Work out the finished part from the listing and answer in its coordinate system (mm). A direction names the side the tool comes from. Give positions to 0.01 mm unless a question says otherwise; leave off trailing zeros. Write each loop counter-clockwise with the first axis right and the second up, starting at its lowest first coordinate (ties: lowest second). Pieces come first, ordered by that corner, then holes.
1) Determine the mould class of faces 1 (the face through (6, 0, 3)), 2 (the face through (0, 3.8, 8)), 3 (the face through (1.5, 0.07, -0.49)) for opening direction X: pulls with the +X half, pulls with the -X half, needs draft (parallel to the pull), parting line crosses it, or undercut.
2) Find section D-D (x = 2.5). Determine the outline of the cut face in (y, z), plus the area to 3 significant figures.
3) Find section B-B (x = 0). Determine the outline of the cut face in (y, z).
4) Given pin 1 Ø1.5 at (y, z) = (2, -1.5) entering from +X; pin 2 Ø3 at (y, z) = (3.5, 0) entering from +X; pin 3 Ø1.2 at (x, z) = (0, 8.5) entering from +Y, each flat-ended and moving along its own axis, determine where each tip first touches the part or whether it passes through.
5) Straight lines are drawn through the part: probe 1 along Y at (x, z) = (2.5, -0.25); probe 2 along X at (y, z) = (5.25, 1.5); probe 3 along Y at (x, z) = (1.5, 6.75). For each, find the intervals that lie inside material, in ascending order.
6) Find section C-C (y = 4). Determine the outline of the cut face in (x, z).
7) A tool of negligible diameter and unlimited length cuts with its end or side. For faces 4 (the face through (4, 0, 6)), 5 (the face through (4.6, 0, -0.5)), 6 (the face through (3.8, 0, 8)), 7 (the face through (-3.8, 0, 8)), 8 (the face through (0, -3.8, 8)), from which of +Z, -Z, +X, -X, +Y, -Y can it reach the whole face along a straight path? Write none if from no direction.
8) Find section A-A (z = 9.25). Determine the outline of the cut face in (x, y), plus the area to 3 significant figures.
```python
from build123d import *

# Parameters (mm, degrees)
BOSS_EXTRU_1_DEPTH      = 6
ESQUISSE2_W             = 7.6
ESQUISSE2_H             = 7.6
BOSS_EXTRU_2_DEPTH      = 4
ENL_V_MAT_EXTRU_1_DEPTH = 0.1
ESQUISSE4_R             = 1.5
ESQUISSE4_R_2           = 0.6
BOSS_EXTRU_4_DEPTH      = 1.2
ESQUISSE5_R             = 0.4
BOSS_EXTRU_5_DEPTH      = 5.2
CONG_1_R                = 0.5


with BuildPart() as part:
    # Esquisse1 → Boss.-Extru.1 (new body)
    with BuildSketch(Plane.XY):
        with BuildLine():
            Line((-5.4, 2.615339366), (-5.4, -2.615339366))
            ThreePointArc((-5.4, -2.615339366), (6, 0), (-5.4, 2.615339366))
        make_face()
    extrude(amount=BOSS_EXTRU_1_DEPTH)

    # Esquisse2 → Boss.-Extru.2 (add)
    with BuildSketch(Plane.XY.offset(6)):
        Rectangle(ESQUISSE2_W, ESQUISSE2_H)
    extrude(amount=BOSS_EXTRU_2_DEPTH)

    # Esquisse3 → Enlèv. mat.-Extru.1 (cut)
    with BuildSketch(Plane(origin=(0, 0, 0), x_dir=(-1, 0, 0), z_dir=(0, 0, -1))):
        with BuildLine():
            Line((4.8, -2.473863375), (4.8, 2.473863375))
            ThreePointArc((4.8, 2.473863375), (-5.4, 0), (4.8, -2.473863375))
        make_face()
    extrude(amount=-ENL_V_MAT_EXTRU_1_DEPTH, mode=Mode.SUBTRACT)

    # Esquisse4 → Boss.-Extru.4 (add)
    with BuildSketch(Plane(origin=(0, 0, 0.1), x_dir=(-1, 0, 0), z_dir=(0, 0, -1))):
        Circle(ESQUISSE4_R)
        with Locations((0, -4)):
            Circle(ESQUISSE4_R_2)
        with Locations((-4, 0)):
            Circle(ESQUISSE4_R_2)
        with Locations((0, 4)):
            Circle(ESQUISSE4_R_2)
        with Locations((4, 0)):
            Circle(ESQUISSE4_R_2)
    extrude(amount=BOSS_EXTRU_4_DEPTH)

    # Esquisse5 → Boss.-Extru.5 (add)
    with BuildSketch(Plane(origin=(0, 0, 0.1), x_dir=(-1, 0, 0), z_dir=(0, 0, -1))):
        with Locations((2.5, -2.5)):
            Circle(ESQUISSE5_R)
        with Locations((-2.5, -2.5)):
            Circle(ESQUISSE5_R)
        with Locations((-2.5, 2.5)):
            Circle(ESQUISSE5_R)
        with Locations((2.5, 2.5)):
            Circle(ESQUISSE5_R)
    extrude(amount=BOSS_EXTRU_5_DEPTH)

    # Congé1
    cong_1_edges = [part.edges().sort_by_distance(p)[0] for p in [
        (3.8, -3.8, 8),
        (3.8, 3.8, 8),
        (-3.8, 3.8, 8),
        (-3.8, -3.8, 8),
    ]]
    fillet(cong_1_edges, radius=CONG_1_R)


solid = part.part
```
Results:
1. face 1: parting line crosses it
1. face 2: needs draft
1. face 3: undercut
2. outline: (-5.45, 0) - (-4.79, 0) - (-4.79, 0.1) - (-2.9, 0.1) - (-2.9, -5.1) - (-2.1, -5.1) - (-2.1, 0.1) - (2.1, 0.1) - (2.1, -5.1) - (2.9, -5.1) - (2.9, 0.1) - (4.79, 0.1) - (4.79, 0) - (5.45, 0) - (5.45, 6) - (3.8, 6) - (3.8, 10) - (-3.8, 10) - (-3.8, 6) - (-5.45, 6) - close
2. area: 103 mm2
3. outline: (-6, 0) - (-5.4, 0) - (-5.4, 0.1) - (-4.6, 0.1) - (-4.6, -1.1) - (-3.4, -1.1) - (-3.4, 0.1) - (-1.5, 0.1) - (-1.5, -1.1) - (1.5, -1.1) - (1.5, 0.1) - (3.4, 0.1) - (3.4, -1.1) - (4.6, -1.1) - (4.6, 0.1) - (5.4, 0.1) - (5.4, 0) - (6, 0) - (6, 6) - (3.8, 6) - (3.8, 10) - (-3.8, 10) - (-3.8, 6) - (-6, 6) - close
4. pin 1: stops at x = 2.9
4. pin 2: stops at x = 5.66
4. pin 3: stops at y = 3.8
5. probe 1: y = -2.9 to -2.1, 2.1 to 2.9
5. probe 2: x = -2.9 to 2.9
5. probe 3: y = -3.8 to 3.8
6. outline: (-4.47, 0) - (-3.63, 0) - (-3.63, 0.1) - (-0.6, 0.1) - (-0.6, -1.1) - (0.6, -1.1) - (0.6, 0.1) - (3.63, 0.1) - (3.63, 0) - (4.47, 0) - (4.47, 6) - (-4.47, 6) - close
7. face 4: +Z
7. face 5: -Z
7. face 6: +Z, +X, +Y, -Y
7. face 7: +Z, -X, +Y, -Y
7. face 8: +Z, +X, -X, -Y
8. outline: (-3.8, -3.3) arc R0.5 ccw to (-3.3, -3.8) - (3.3, -3.8) arc R0.5 ccw to (3.8, -3.3) - (3.8, 3.3) arc R0.5 ccw to (3.3, 3.8) - (-3.3, 3.8) arc R0.5 ccw to (-3.8, 3.3) - close
8. area: 57.5 mm2
